Build history of the part. All positions in model axes, mm. A direction names the side the tool comes from. Give positions to 0.01 mm unless a question says otherwise; leave off trailing zeros. Loops run counter-clockwise (first coordinate to the right, second up) from the corner with the lowest first, then second, coordinate; pieces in that order, holes last. Notation, with made-up numbers: M -28.5,63.5 L -19.5,63.5 A35 cw -19.5,100.5 Z; hole C -32.5,-3 d3. An arc over 180 degrees is marked long. Put each result on its own line as item: value.
Autodesk Inventor part; units mm, degrees
ref_plane "YZ Plane" through (0, 0, 0) normal (1, 0, 0) x (0, 1, 0)
ref_plane "XZ Plane" through (0, 0, 0) normal (0, 1, 0) x (-1, 0, 0)
ref_plane "XY Plane" through (0, 0, 0) normal (0, 0, 1) x (1, 0, 0)
sketch "Boceto1" plane through (0, 0, 0) normal (0, 0, 1) x (1, 0, 0)
  circle A0 centre (0, 0) radius 2.1
  line L0 (-12, 0) -> (12, 0)
  line L1 (0, 12) -> (0, -12)
  line L2 (0, 3.9) -> (-2.8387, 3.9)
  line L3 (-2.8387, 3.9) -> (-5.5, 6.555)
  line L4 (-5.5, 6.555) -> (-5.5, 8.195)
  line L5 (-5.5, 8.195) -> (-3.125, 8.195)
  line L6 (-3.125, 8.545) -> (-4.58, 10)
  line L7 (-4.58, 10) -> (-10, 10)
  line L8 (-10, 10) -> (-10, 4.58)
  line L9 (-10, 4.58) -> (-8.5415, 3.125)
  line L10 (-8.1915, 3.125) -> (-8.1915, 5.4852)
  line L11 (-8.1915, 5.4852) -> (-6.5515, 5.4852)
  line L12 (-6.5515, 5.4852) -> (-3.9, 2.84)
  line L13 (-3.9, 2.84) -> (-3.9, 0)
  line L14 (3.125, 8.545) -> (4.58, 10)
  line L15 (5.5, 8.195) -> (3.125, 8.195)
  line L16 (5.5, 6.555) -> (5.5, 8.195)
  line L17 (2.8387, 3.9) -> (5.5, 6.555)
  line L18 (0, 3.9) -> (2.8387, 3.9)
  line L19 (3.9, 2.84) -> (3.9, 0)
  line L20 (-10, -10) -> (-10, -4.58)
  line L21 (-4.58, -10) -> (-10, -10)
  line L22 (-3.125, -8.545) -> (-4.58, -10)
  line L23 (-5.5, -8.195) -> (-3.125, -8.195)
  line L24 (-5.5, -6.555) -> (-5.5, -8.195)
  line L25 (-2.8387, -3.9) -> (-5.5, -6.555)
  line L26 (0, -3.9) -> (-2.8387, -3.9)
  line L27 (0, -3.9) -> (2.8387, -3.9)
  line L28 (2.8387, -3.9) -> (5.5, -6.555)
  line L29 (5.5, -6.555) -> (5.5, -8.195)
  line L30 (5.5, -8.195) -> (3.125, -8.195)
  line L31 (3.125, -8.545) -> (4.58, -10)
  line L32 (7.3, -6.2319) -> (3.9, -2.84)
  line L33 (3.9, -2.84) -> (3.9, 0)
  line L34 (-3.9, -2.84) -> (-3.9, 0)
  line L35 (-6.5515, -5.4852) -> (-3.9, -2.84)
  line L36 (-8.1915, -5.4852) -> (-6.5515, -5.4852)
  line L37 (-8.1915, -3.125) -> (-8.1915, -5.4852)
  line L38 (-10, -4.58) -> (-8.5415, -3.125)
  line L39 (-3.125, 8.195) -> (-3.125, 8.545)
  line L40 (-8.1915, 3.125) -> (-8.5415, 3.125)
  line L41 (3.125, 8.195) -> (3.125, 8.545)
  line L42 (-8.1915, -3.125) -> (-8.5415, -3.125)
  line L43 (-3.125, -8.195) -> (-3.125, -8.545)
  line L44 (3.125, -8.195) -> (3.125, -8.545)
  line L45 (10, 12) -> (10, -12)
  line L46 (16.875, 8.195) -> (16.875, 8.545)
  line L47 (14.5, 8.195) -> (16.875, 8.195)
  line L48 (14.5, 6.555) -> (14.5, 8.195)
  line L49 (16.875, 8.545) -> (15.42, 10)
  line L50 (17.1613, 3.9) -> (14.5, 6.555)
  line L51 (20, 3.9) -> (17.1613, 3.9)
  line L52 (32, 0) -> (8, 0)
  line L53 (20, 3.9) -> (22.8387, 3.9)
  line L54 (23.125, 8.195) -> (23.125, 8.545)
  circle A1 centre (20, 0) radius 2.1
  line L55 (23.9, -2.84) -> (23.9, 0)
  line L56 (26.5515, -5.4852) -> (23.9, -2.84)
  line L57 (28.1915, -5.4852) -> (26.5515, -5.4852)
  line L58 (24.58, -10) -> (30, -10)
  line L59 (30, -10) -> (30, -4.58)
  line L60 (28.1915, -3.125) -> (28.1915, -5.4852)
  line L61 (30, -4.58) -> (28.5415, -3.125)
  line L62 (28.1915, -3.125) -> (28.5415, -3.125)
  line L63 (22.8387, -3.9) -> (25.5, -6.555)
  line L64 (25.5, -8.195) -> (23.125, -8.195)
  line L65 (23.125, -8.195) -> (23.125, -8.545)
  line L66 (23.125, -8.545) -> (24.58, -10)
  line L67 (20, -3.9) -> (22.8387, -3.9)
  line L68 (20, -3.9) -> (17.1613, -3.9)
  line L69 (16.875, -8.195) -> (16.875, -8.545)
  line L70 (25.5, -6.555) -> (25.5, -8.195)
  line L71 (12.7, -6.2319) -> (16.1, -2.84)
  line L72 (17.1613, -3.9) -> (14.5, -6.555)
  line L73 (14.5, -8.195) -> (16.875, -8.195)
  line L74 (16.875, -8.545) -> (15.42, -10)
  line L75 (14.5, -6.555) -> (14.5, -8.195)
  line L76 (20, 12) -> (20, -12)
  line L77 (22.8387, 3.9) -> (25.5, 6.555)
  line L78 (25.5, 6.555) -> (25.5, 8.195)
  line L79 (25.5, 8.195) -> (23.125, 8.195)
  line L80 (23.125, 8.545) -> (24.58, 10)
  line L81 (24.58, 10) -> (30, 10)
  line L82 (30, 10) -> (30, 4.58)
  line L83 (30, 4.58) -> (28.5415, 3.125)
  line L84 (28.1915, 3.125) -> (28.1915, 5.4852)
  line L85 (28.1915, 5.4852) -> (26.5515, 5.4852)
  line L86 (26.5515, 5.4852) -> (23.9, 2.84)
  line L87 (23.9, 2.84) -> (23.9, 0)
  line L88 (28.1915, 3.125) -> (28.5415, 3.125)
  line L89 (16.1, 2.84) -> (16.1, 0)
  line L90 (16.1, -2.84) -> (16.1, 0)
  line L91 (7.3, -6.2319) -> (7.3, -8.195)
  line L92 (7.3, -8.195) -> (12.7, -8.195)
  line L93 (12.7, -8.195) -> (12.7, -6.2319)
  line L94 (4.58, 10) -> (15.42, 10)
  line L95 (4.58, -10) -> (15.42, -10)
  line L96 (3.9, 2.84) -> (7.3, 6.2319)
  line L97 (7.3, 6.2319) -> (7.3, 8.195)
  line L98 (7.3, 8.195) -> (12.7, 8.195)
  line L99 (12.7, 8.195) -> (12.7, 6.2319)
  line L100 (16.1, 2.84) -> (12.7, 6.2319)
  point P0 (10, 0)
  dimension "d0" = 4.2
  dimension "d1" = 24
  dimension "d2" = 24
  dimension "d3" = 90
  dimension "d6" = 20
  dimension "d7" = 1.5
  dimension "d8" = 1.64
  dimension "d9" = 1.64
  dimension "d10" = 7.8
  dimension "d11" = 11
  dimension "d12" = 9.16
  dimension "d14" = 6.25
  dimension "d15" = 6.25
  dimension "d16" = 0.35
  dimension "d17" = 7.8
  dimension "d18" = 0.35
  dimension "d20" = 24
  dimension "d24" = 12.2
  dimension "d25" = 9.16
  dimension "d26" = 5.68
  dimension "d31" = 5.4
  dimension "d32" = 5.4
  dimension "d34" = 40
extrude "Extrusión1" add sketch "Boceto1" against normal blind 200 contours L0 L33 L32 L91 L92 L45 L95 L31 L44 L30 L29 L28 L27 L1 A0 | A0 L1 L18 L17 L16 L15 L41 L14 L94 L45 L98 L97 L96 L19 L0 | A0 L0 L13 L12 L11 L10 L40 L9 L8 L7 L6 L39 L5 L4 L3 L2 L1 | L1 L26 L25 L24 L23 L43 L22 L21 L20 L38 L42 L37 L36 L35 L34 L0 A0 | L45 L94 L49 L46 L47 L48 L50 L51 L76 A1 L52 L89 L100 L99 L98 | L92 L93 L71 L90 L52 A1 L76 L68 L72 L75 L73 L69 L74 L95 L45 | L76 L53 L77 L78 L79 L54 L80 L81 L82 L83 L88 L84 L85 L86 L87 L52 A1 | A1 L52 L55 L56 L57 L60 L62 L61 L59 L58 L66 L65 L64 L70 L63 L67 L76
fillet "Empalme1" radius 0.5 4 edges at (-10, 10, -100) (30, 10, -100) (30, -10, -100) (-10, -10, -100)
properties part number "Perfil2040" material "Aluminio 6061"
Q1. Drop flat-ended pins along their axis: pin 1 Ø2 at (y, z) = (-2, -146.5) entering from +X; pin 2 Ø2.5 at (x, y) = (0, 0) entering from +Z; pin 3 Ø3 at (x, z) = (-0.5, -114.5) entering from +Y; pin 4 Ø1.7 at (y, z) = (0, -62.5) entering from -X. Give the stop position or say it passes through.
Here are the results:
pin 1: x = 24.06
pin 2: through
pin 3: y = 3.9
pin 4: x = -3.9
Q2. Slice it at D-D (z = -72). State how many separate pieces and enclosed holes the cut face has, and give its area (3 significant figures).
Here are the results:
separate pieces: 1
enclosed holes: 3
area: 301 mm²
Q3. Tool access for faces 5 (the flat face through (0, 3.9, -99)), 6 (the flat face through (14.376, -4.56, -98.6)), 7 (the flat face through (23.9, 0, -99)): list every direction of +Z, -Z, +X, -X, +Y, -Y with a clear straight run to the whole face (end or side of a thin tool).
Here are the results:
face 5: +Z, -Z, +Y
face 6: +Z, -Z
face 7: +Z, -Z, +X
Q4. Slice it at A-A (y = 0). List the corners of the cut face in (x, z).
Here are the results:
outline: M -3.9,-200 L -2.1,-200 L -2.1,0 L -3.9,0 Z; M 2.1,-200 L 3.9,-200 L 3.9,0 L 2.1,0 Z; M 16.1,-200 L 17.9,-200 L 17.9,0 L 16.1,0 Z; M 22.1,-200 L 23.9,-200 L 23.9,0 L 22.1,0 Z
Q5. Mould opens along X. For faces 1 (the flat face through (-3.9, 0, -99)), 2 (the flat face through (20, 3.9, -99)), 3 (the flat face through (5, 5, 0)), 4 (the flat face through (5.576, 4.512, -98.6)) say: pulls with the +X half, pulls with the -X half, needs draft (parallel to the pull), parting line crosses it, or undercut.
Here are the results:
face 1: pulls with the -X half
face 2: undercut
face 3: needs draft
face 4: undercut
Q6. Slice it at C-C (x = 20). List the corners of the cut face in (y, z), and give its area (3 significant figures).
Here are the results:
outline: M -3.9,-200 L -2.1,-200 L -2.1,0 L -3.9,0 Z; M 2.1,-200 L 3.9,-200 L 3.9,0 L 2.1,0 Z
area: 720 mm²
Q7. Slice it at B-B (x = 10). List the corners of the cut face in (y, z) (3 decimals).
Here are the results:
outline: M -10,-200 L -8.195,-200 L -8.195,0 L -10,0 Z; M 8.195,-200 L 10,-200 L 10,0 L 8.195,0 Z
Q8. Probe line 1 (X direction, y = 7.5, z = -176); line 2 (X direction, y = 0, z = -153.5); line 3 (Y direction, x = 0, z = -153). List the from-to ranges inside material, lowest first. Write a range as from..to.
Here are the results:
line 1: -10..-5.5, 5.5..7.3, 12.7..14.5, 25.5..30
line 2: -3.9..-2.1, 2.1..3.9, 16.1..17.9, 22.1..23.9
line 3: -3.9..-2.1, 2.1..3.9
